from build123d import *

# Parameters (mm, degrees)
BOSS_EXTRUDE1_DEPTH = 19
SKETCH2_3_R         = 2.1
BOSS_EXTRUDE2_DEPTH = 2
BOSS_EXTRUDE3_DEPTH = 4
SKETCH3_R           = 4.5
BOSS_EXTRUDE4_DEPTH = 1.5
SKETCH5_R           = 2.5
BOSS_EXTRUDE5_DEPTH = 10
CUT_EXTRUDE1_START  = -6
CUT_EXTRUDE1_DEPTH  = 6


with BuildPart() as part:
    # Sketch2 → Boss-Extrude1 (new body)
    with BuildSketch(Plane.XY):
        with BuildLine():
            ThreePointArc((13.555441712, 3.5), (-1.764060095, 13.888415748), (-14, 0))
            Line((-14, 0), (14, 0))
            ThreePointArc((14, 0), (13.888415748, 1.764060095), (13.555441712, 3.5))
        make_face()
        with BuildLine():
            Line((14, 0), (-14, 0))
            ThreePointArc((-14, 0), (-12.210651088, -6.848357467), (-7.3, -11.94612908))
            ThreePointArc((-7.3, -11.94612908), (0, -14), (7.3, -11.94612908))
            ThreePointArc((7.3, -11.94612908), (11.250406053, -8.332368429), (13.555441712, -3.5))
            ThreePointArc((13.555441712, -3.5), (13.888415748, -1.764060095), (14, 0))
        make_face()
    extrude(amount=BOSS_EXTRUDE1_DEPTH)

    # Sketch2_3 → Boss-Extrude2 (add)
    with BuildSketch(Plane.XY):
        with BuildLine():
            ThreePointArc((17.5, -3.5), (21, 0), (17.5, 3.5))
            Line((17.5, 3.5), (13.555441712, 3.5))
            ThreePointArc((13.555441712, 3.5), (13.888415748, 1.764060095), (14, 0))
            ThreePointArc((14, 0), (13.888415748, -1.764060095), (13.555441712, -3.5))
            Line((13.555441712, -3.5), (17.5, -3.5))
        make_face()
        with Locations((17.5, 0)):
            Circle(SKETCH2_3_R, mode=Mode.SUBTRACT)
    boss_extrude2 = extrude(amount=BOSS_EXTRUDE2_DEPTH)

    # Mirror1: Boss-Extrude2 across plane
    add(boss_extrude2.mirror(Plane(origin=(0, 0, 0), x_dir=(0, 0, 1), z_dir=(1, 0, 0))))

    # Sketch2_4 → Boss-Extrude3 (add)
    with BuildSketch(Plane.XY):
        with BuildLine():
            ThreePointArc((7.3, -11.94612908), (0, -14), (-7.3, -11.94612908))
            Line((-7.3, -11.94612908), (-7.3, -17))
            Line((-7.3, -17), (7.3, -17))
            Line((7.3, -17), (7.3, -11.94612908))
        make_face()
    extrude(amount=BOSS_EXTRUDE3_DEPTH)

    # Sketch3 → Boss-Extrude4 (add)
    with BuildSketch(Plane.XY):
        with Locations((0, 8)):
            Circle(SKETCH3_R)
    extrude(amount=-BOSS_EXTRUDE4_DEPTH)

    # Sketch5 → Boss-Extrude5 (add)
    with BuildSketch(Plane.XY):
        with Locations((0, 8)):
            Circle(SKETCH5_R)
    extrude(amount=-BOSS_EXTRUDE5_DEPTH)

    # Sketch7 → Cut-Extrude1 (cut)
    with BuildSketch(Plane(origin=(0, 0, -10), x_dir=(-1, 0, 0), z_dir=(0, 0, -1)).offset(CUT_EXTRUDE1_START)):
        with BuildLine():
            ThreePointArc((2, 9.5), (0, 10.5), (-2, 9.5))
            Line((-2, 9.5), (2, 9.5))
        make_face()
        with BuildLine():
            ThreePointArc((-2, 6.5), (0, 5.5), (2, 6.5))
            Line((2, 6.5), (-2, 6.5))
        make_face()
    extrude(amount=CUT_EXTRUDE1_DEPTH, mode=Mode.SUBTRACT)


solid = part.part
For this review, take the finished solid that the model builds, in its own axes (mm). A direction names the side the tool comes from. Coordinates: 2 decimals unless noted, no trailing zeros. Write each loop counter-clockwise with the first axis right and the second up, starting at its lowest first coordinate (ties: lowest second). Pieces come first, ordered by that corner, then holes. Notation, with made-up numbers: (69.5, -17.75) -> (116.5, -17.75) arc R16 ccw to (116.5, -11.75) -> close; hole circle Ø11 at (23.5, -24.75). An arc over 180 degrees is marked (long way). Write each question's results on one line, items separated by ' | '. Start each with the question number.
1) For faces 1 (the face through (2.385, 8.751, -4.746)), 2 (the face through (0, 6.5, -7)), 3 (the face through (-16, -3.5, 1)), 4 (the face through (0, 10, -4)), 5 (the face through (-16, 3.5, 1)), list the 3-axis set-ups (+Z, -Z, +X, -X, +Y, -Y) from which the entire face can be reached by the end or side of a thin tool; tool diameter is ignored.
2) Consider section C-C (x = 0). Write out the cut boundary in (y, z).
3) The part is to be moulded in two halves that separate along X. For faces 6 (the face through (0, 6, -4)), 7 (the face through (-19.503, 0.631, 0.986)), 8 (the face through (7.3, -15, 2)), 9 (the face through (-21, 0, 1)), say which applies: +X half, -X half, draft (parallel to the pull), parting line (faces both ways), or undercut.
4) Consider section A-A (z = 1.5). Write out the cut boundary in (x, y), plus the area to 3 significant figures.
5) Consider section B-B (x = -17). Write out the cut boundary in (y, z).
6) Insertion check: pin 1 (4.5 mm diameter, centred on y = -15.5, z = 3, fed in from +X); pin 2 (4 mm diameter, centred on y = 2, z = -1.5, fed in from +X); pin 3 (1 mm diameter, centred on x = -15.5, z = 0.5, fed in from +Y); pin 4 (4 mm diameter, centred on x = -17.5, y = 0, fed in from -Z). Each pin has a flat end and moves straight along its axis. Give the tip position at first contact, or say it passes through.
7) Consider section D-D (y = -0.5). Write out the cut boundary in (x, z), plus the area to 3 significant figures.
8) Wall thickness on L1, parallel to Y at x = -17.5, z = 0.65; L2, parallel to Z at x = 10.5, y = 8; L3, parallel to X at y = 8, z = -5.75: over which ranges is each line inside the solid? List them lowest first. Write a range as [from, to].
Geometry says:
1) face 1: -Z | face 2: -Z, +X, -X, -Y | face 3: +Z, -Z, -X, -Y | face 4: -Z, +X, -X, +Y | face 5: +Z, -Z, -X, +Y
2) outline: (-17, 0) -> (3.5, 0) -> (3.5, -1.5) -> (5.5, -1.5) -> (5.5, -4) -> (6.5, -4) -> (6.5, -10) -> (9.5, -10) -> (9.5, -4) -> (10.5, -4) -> (10.5, -1.5) -> (12.5, -1.5) -> (12.5, 0) -> (14, 0) -> (14, 19) -> (-14, 19) -> (-14, 4) -> (-17, 4) -> close
3) face 6: draft | face 7: undercut | face 8: +X half | face 9: -X half
4) outline: (-17.5, -3.5) -> (-13.56, -3.5) arc R14 ccw to (-7.3, -11.95) -> (-7.3, -17) -> (7.3, -17) -> (7.3, -11.95) arc R14 ccw to (13.56, -3.5) -> (17.5, -3.5) arc R3.5 ccw to (17.5, 3.5) -> (13.56, 3.5) arc R14 ccw to (-13.56, 3.5) -> (-17.5, 3.5) arc R3.5 ccw to start; hole circle Ø4.2 at (-17.5, 0); hole circle Ø4.2 at (17.5, 0) | area: 731 mm^2
5) outline: (-3.5, 0) -> (-2.04, 0) -> (-2.04, 2) -> (-3.5, 2) -> close; (2.04, 0) -> (3.5, 0) -> (3.5, 2) -> (2.04, 2) -> close
6) pin 1: x = 7.3 | pin 2: x = 20.93 | pin 3: y = 3.5 | pin 4: through
7) outline: (-20.96, 0) -> (-19.54, 0) -> (-19.54, 2) -> (-20.96, 2) -> close; (-15.46, 0) -> (15.46, 0) -> (15.46, 2) -> (13.99, 2) -> (13.99, 19) -> (-13.99, 19) -> (-13.99, 2) -> (-15.46, 2) -> close; (19.54, 0) -> (20.96, 0) -> (20.96, 2) -> (19.54, 2) -> close | area: 543 mm^2
8) L1: [-3.5, -2.1], [2.1, 3.5] | L2: [0, 19] | L3: [-2.5, 2.5]
